Could you check a few things on this model? Use its own coordinates, in mm. A direction names the side the tool comes from. Coordinates: 2 decimals unless noted, no trailing zeros. Write each loop counter-clockwise with the first axis right and the second up, starting at its lowest first coordinate (ties: lowest second). Pieces come first, ordered by that corner, then holes.
Item 1: If I drill on probe 1 along Z at (x, y) = (0, 0.65) (3 decimals); probe 2 along Z at (x, y) = (-6, 1.25) (3 decimals); probe 3 along X at (y, z) = (0.95, 10.5) (3 decimals), over which ranges is the centre line in solid material (lowest first)?
Item 2: I want a section at B-B on z = 9.5. Please give me the cut outline in (x, y) (3 decimals), then the cut area to 3 significant figures.
Item 3: Thinking about a two-plate mould opening in X: for faces 4 (the flat face through (15.875, 1, 0)), 5 (the flat face through (14, 1, 12.7)), 6 (the flat face through (-8, 1, -9.2)), which applies, +X half, -X half, draft (parallel to the pull), parting line (faces both ways), or undercut?
Item 4: I want a section at A-A on x = 0. Please give me the cut outline in (y, z) (3 decimals).
Item 5: I want a section at C-C on x = 9.5. Please give me the cut outline in (y, z) (3 decimals).
Item 6: For P1, Ø5, axis at x = -9.5, z = 1.5, coming from the -Y side; P2, Ø1, axis at x = -11, y = 0.5, coming from the +Z side, each with a flat end and sliding along its axis, tell me the tip position at first contact or that it passes through.
Item 7: Which directions (+Z, -Z, +X, -X, +Y, -Y) give clear straight access to the entire face, cutting with the end or side of a thin tool? Please do faces 1 (the flat face through (-4.075, 1, 11)), 2 (the flat face through (0, 2, -3)), 3 (the cylindrical face through (4.45, 0.99, -2.93)).
Item 8: I want a section at D-D on z = -8.5. Please give me the cut outline in (x, y) (1 decimal), then the cut area to 3 significant figures.
from build123d import *

# Parameters (mm, degrees)
F1_W     = 31.75
F1_H     = 25.4
F2_DEPTH = 2
F3_R     = 3.5
F3_R_2   = 1.575
F5_DEPTH = 2.001


with BuildPart() as f2:
    # F1 (on Front) → F2 (new body)
    with BuildSketch(Plane.XZ):
        Rectangle(F1_W, F1_H)
    extrude(amount=-F2_DEPTH)

    # F3 (on face) + F4 (on face) → F5 (cut, through all)
    with BuildSketch(Plane.XZ):
        with Locations((0, 1.5)):
            Circle(F3_R)
        with Locations((-9.5, 1.5)):
            Circle(F3_R_2)
        with Locations((9.5, 1.5)):
            Circle(F3_R_2)
        with Locations((0, 9.5)):
            Circle(F3_R_2)
        with Locations((0, -6.5)):
            Circle(F3_R_2)
    with BuildSketch(Plane.XZ):
        with BuildLine():
            Line((-4.075, -7.95), (-4.075, -3.825))
            ThreePointArc((-4.075, -3.825), (-4.4411165235, -2.9411165235), (-5.325, -2.575))
            Line((-5.325, -2.575), (-11.125, -2.575))
            ThreePointArc((-11.125, -2.575), (-12.0088834765, -2.9411165235), (-12.375, -3.825))
            Line((-12.375, -3.825), (-12.375, -7.95))
            ThreePointArc((-12.375, -7.95), (-12.0088834765, -8.8338834765), (-11.125, -9.2))
            Line((-11.125, -9.2), (-5.325, -9.2))
            ThreePointArc((-5.325, -9.2), (-4.4411165235, -8.8338834765), (-4.075, -7.95))
        make_face()
        with BuildLine():
            ThreePointArc((5.325, -2.575), (4.4411165235, -2.9411165235), (4.075, -3.825))
            Line((4.075, -3.825), (4.075, -7.95))
            ThreePointArc((4.075, -7.95), (4.4411165235, -8.8338834765), (5.325, -9.2))
            Line((5.325, -9.2), (11.125, -9.2))
            ThreePointArc((11.125, -9.2), (12.0088834765, -8.8338834765), (12.375, -7.95))
            Line((12.375, -7.95), (12.375, -3.825))
            ThreePointArc((12.375, -3.825), (12.0088834765, -2.9411165235), (11.125, -2.575))
            Line((11.125, -2.575), (5.325, -2.575))
        make_face()
        with BuildLine():
            Line((-4.075, 12.7), (-12.375, 12.7))
            Line((-12.375, 12.7), (-12.375, 8.95))
            ThreePointArc((-12.375, 8.95), (-12.0088834765, 8.0661165235), (-11.125, 7.7))
            Line((-11.125, 7.7), (-5.325, 7.7))
            ThreePointArc((-5.325, 7.7), (-4.4411165235, 8.0661165235), (-4.075, 8.95))
            Line((-4.075, 8.95), (-4.075, 12.7))
        make_face()
        with BuildLine():
            Line((4.075, 12.7), (4.075, 8.95))
            ThreePointArc((4.075, 8.95), (4.4411165235, 8.0661165235), (5.325, 7.7))
            Line((5.325, 7.7), (11.125, 7.7))
            ThreePointArc((11.125, 7.7), (12.0088834765, 8.0661165235), (12.375, 8.95))
            Line((12.375, 8.95), (12.375, 12.7))
            Line((12.375, 12.7), (4.075, 12.7))
        make_face()
    extrude(amount=-F5_DEPTH, mode=Mode.SUBTRACT)


solid = f2.part
Response values:
1. probe 1: z = -12.7 to -8.075, -4.925 to -2, 5 to 7.925, 11.075 to 12.7
1. probe 2: z = -12.7 to -9.2, -2.575 to 7.7
1. probe 3: x = -15.875 to -12.375, -4.075 to -1.217, 1.217 to 4.075, 12.375 to 15.875
2. outline: (-15.875, 0) - (-12.375, 0) - (-12.375, 2) - (-15.875, 2) - close; (-4.075, 0) - (-1.575, 0) - (-1.575, 2) - (-4.075, 2) - close; (1.575, 0) - (4.075, 0) - (4.075, 2) - (1.575, 2) - close; (12.375, 0) - (15.875, 0) - (15.875, 2) - (12.375, 2) - close
2. area: 24.0 mm2
3. face 4: +X half
3. face 5: draft
3. face 6: undercut
4. outline: (0, -12.7) - (2, -12.7) - (2, -8.075) - (0, -8.075) - close; (0, -4.925) - (2, -4.925) - (2, -2) - (0, -2) - close; (0, 5) - (2, 5) - (2, 7.925) - (0, 7.925) - close; (0, 11.075) - (2, 11.075) - (2, 12.7) - (0, 12.7) - close
5. outline: (0, -12.7) - (2, -12.7) - (2, -9.2) - (0, -9.2) - close; (0, -2.575) - (2, -2.575) - (2, -0.075) - (0, -0.075) - close; (0, 3.075) - (2, 3.075) - (2, 7.7) - (0, 7.7) - close
6. P1: stops at y = 0
6. P2: stops at z = 7.76
7. face 1: +Z, +Y, -Y
7. face 2: +Z, -Z, +X, -X, +Y
7. face 3: +Y, -Y
8. outline: (-15.9, 0) - (-12.2, 0) - (-12.2, 2) - (-15.9, 2) - close; (-4.2, 0) - (4.2, 0) - (4.2, 2) - (-4.2, 2) - close; (12.2, 0) - (15.9, 0) - (15.9, 2) - (12.2, 2) - close
8. area: 31.3 mm2
